Here's the drawing with two shaded views (mm, measured from the low corner). I have some questions. A direction names the side the tool comes from. Coordinates: 2 decimals unless noted, no trailing zeros. Order: outer loops, then holes, each group sorted by start corner. A loop starts at its lowest first (then second) coordinate and runs counter-clockwise, first axis right, second up. Notation, with made-up numbers: (-5.5, 32) - (-0.5, 32) arc R29 ccw to (-0.5, 52) - close; hole circle Ø2 at (82, 0.5). An arc over 180 degrees is marked (long way). Answer as a JSON object with one key per item and string values. Group by question number.
(1) Will these pins go through, and if not, where does the flat tip stop? P1, Ø3, axis at x = 3, z = 3.5, coming from the -Y side; P2, Ø2.5, axis at y = 3, z = 3, coming from the -X side; P3, Ø1.9, axis at x = 2.5, z = 1.5, coming from the +Y side; P4, Ø2, axis at y = 6, z = 4, coming from the +X side.
(2) Imagine slicing it at D-D, the plane y = 11. Write out the boundary of the cut face in (x, z), and give its area (3 significant figures).
(3) Imagine slicing it at A-A, the plane z = 3.5. Write out the boundary of the cut face in (x, y).
(4) Imagine slicing it at C-C, the plane x = 16.5. Write out the boundary of the cut face in (y, z).
(5) Imagine slicing it at B-B, the plane x = 7.5. Write out the boundary of the cut face in (y, z), and give its area (3 significant figures).
(6) Please list where these lines run through material, in increasing order: probe 1 along Y at (x, z) = (7.5, 5.25); probe 2 along Y at (x, z) = (6.75, 3); probe 3 along Y at (x, z) = (15.75, 4.75).
(7) Which directions (+Z, -Z, +X, -X, +Y, -Y) give clear straight access to the entire face, cutting with the end or side of a thin tool? Please do the marked faces 1, 2 and 3.
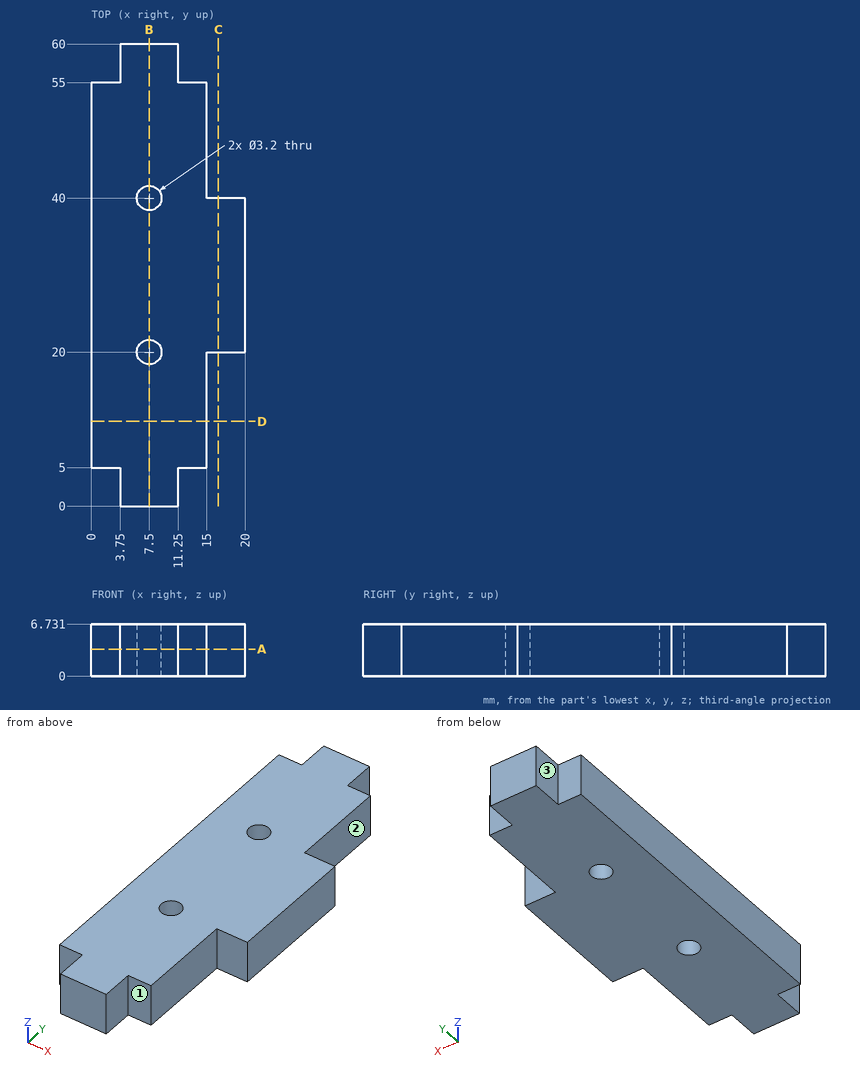
Result set:
{
 "1": {"P1": "stops at y = 0", "P2": "stops at x = 3.75", "P3": "stops at y = 55", "P4": "stops at x = 15"},
 "2": {"outline": "(0, 0) - (15, 0) - (15, 6.73) - (0, 6.73) - close", "area": "101 mm^2"},
 "3": {"outline": "(0, 5) - (3.75, 5) - (3.75, 0) - (11.25, 0) - (11.25, 5) - (15, 5) - (15, 20) - (20, 20) - (20, 40) - (15, 40) - (15, 55) - (11.25, 55) - (11.25, 60) - (3.75, 60) - (3.75, 55) - (0, 55) - close; hole circle Ø3.2 at (7.5, 20); hole circle Ø3.2 at (7.5, 40)"},
 "4": {"outline": "(20, 0) - (40, 0) - (40, 6.73) - (20, 6.73) - close"},
 "5": {"outline": "(0, 0) - (18.4, 0) - (18.4, 6.73) - (0, 6.73) - close; (21.6, 0) - (38.4, 0) - (38.4, 6.73) - (21.6, 6.73) - close; (41.6, 0) - (60, 0) - (60, 6.73) - (41.6, 6.73) - close", "area": "361 mm^2"},
 "6": {"probe 1": "y = 0 to 18.4, 21.6 to 38.4, 41.6 to 60", "probe 2": "y = 0 to 18.59, 21.41 to 38.59, 41.41 to 60", "probe 3": "y = 20 to 40"},
 "7": {"face 1": "+Z, -Z, +X, -Y", "face 2": "+Z, -Z, +X, +Y", "face 3": "+Z, -Z, -X, +Y"}
}
